Autodesk Inventor part; units mm, degrees
ref_plane "YZ Plane" through (0, 0, 0) normal (1, 0, 0) x (0, 1, 0)
ref_plane "XZ Plane" through (0, 0, 0) normal (0, 1, 0) x (-1, 0, 0)
ref_plane "XY Plane" through (0, 0, 0) normal (0, 0, 1) x (1, 0, 0)
sketch "Sketch1" plane through (0, 0, 0) normal (0, 0, 1) x (1, 0, 0)
  circle A0 centre (0, 0) radius 31.5
  circle A1 centre (0, 0) radius 36.5
  dimension "d0" = 63
  dimension "d1" = 5
extrude "Extrusion1" add sketch "Sketch1" along normal blind 60
sketch "Sketch3" plane through (0, 0, 60) normal (0, 0, 1) x (1, 0, 0)
  circle A0 centre (0, 0) radius 31.5
  circle A1 centre (0, 0) radius 36.5
  circle A2 centre (0, 0) radius 32.5
  dimension "d4" = 65
extrude "Extrusion2" cut sketch "Sketch3" against normal blind 29 contours A2
sketch "Sketch4" plane through (0, 0, 0) normal (0, 0, -1) x (-1, 0, 0)
  circle A0 centre (0, 0) radius 31.5
  circle A1 centre (0, 0) radius 36.5
  circle A2 centre (0, 0) radius 32.5
  dimension "d7" = 65
extrude "Extrusion3" cut sketch "Sketch4" against normal blind 29 contours A2
properties part number "coupler_2in" material "PVC-Piping"
Geometry: final body of the model. Coordinates: model frame, mm. A direction names the side the tool comes from. Give positions to 0.01 mm unless a question says otherwise; leave off trailing zeros. Write each loop counter-clockwise with the first axis right and the second up, starting at its lowest first coordinate (ties: lowest second). Pieces come first, ordered by that corner, then holes.
1. Pin query (flat end, axial travel): P1, Ø10, axis at y = 10.5, z = 22.5, coming from the +X side; P2, Ø1.5, axis at x = -3.5, z = 18.5, coming from the +Y side; P3, Ø2, axis at y = -26, z = 39.5, coming from the -X side; P4, Ø4, axis at x = 27.5, y = -10, coming from the -Z side. Return the tip coordinate at first contact, or that it passes through.
2. Draft query along X for faces 1 (the flat face through (-33, -3, 60)), 2 (the cylindrical face through (31, 9.76, 45.7)), 3 (the cylindrical face through (-7.912, 35.632, 29.58)). Return one class per face: released by +X, released by -X, zero draft, split by the parting line, or undercut.
3. Line query: probe 1 along Y at (x, z) = (0, 48); probe 2 along Y at (x, z) = (0, 30); probe 3 along X at (y, z) = (8.5, 42). Output: solid intervals per line, ascending.
4. Reachability of faces 4 (the cylindrical face through (-4.101, -31.232, 29.986)), 5 (the flat face through (-17, 27, 31)), 6 (the cylindrical face through (-31, 9.76, 14.3)) from +Z, -Z, +X, -X, +Y, -Y: full face, straight path, thin tool, end or side. Return the list, or none.
5. Section query A-A, the plane y = 0. Return loops of the section in (x, z), then the cut area to 3 significant figures.
6. Section query C-C, the plane z = 52. Return loops of the section in (x, y).
Computed:
1. P1: stops at x = 36.08
1. P2: stops at y = 36.4
1. P3: stops at x = -26.59
1. P4: passes through
2. face 1: zero draft
2. face 2: undercut
2. face 3: split by the parting line
3. probe 1: y = -36.5 to -32.5, 32.5 to 36.5
3. probe 2: y = -36.5 to -31.5, 31.5 to 36.5
3. probe 3: x = -35.5 to -31.37, 31.37 to 35.5
4. face 4: +Z, -Z
4. face 5: +Z
4. face 6: -Z
5. outline: (-36.5, 0) - (-32.5, 0) - (-32.5, 29) - (-31.5, 29) - (-31.5, 31) - (-32.5, 31) - (-32.5, 60) - (-36.5, 60) - close; (31.5, 29) - (32.5, 29) - (32.5, 0) - (36.5, 0) - (36.5, 60) - (32.5, 60) - (32.5, 31) - (31.5, 31) - close
5. area: 484 mm2
6. outline: circle Ø73 at (0, 0); hole circle Ø65 at (0, 0)
